Here's how the part is built. I have some questions about the finished solid (model axes, mm). A direction names the side the tool comes from. Round coordinates to 2 decimals unless told otherwise and drop trailing zeros. Order: outer loops, then holes, each group sorted by start corner. A loop starts at its lowest first (then second) coordinate and runs counter-clockwise, first axis right, second up. Notation, with made-up numbers: (-16, 19) -> (6, 19) arc R24 ccw to (6, 34) -> close; hole circle Ø11 at (-26, 69). An arc over 180 degrees is marked (long way). Use a Markdown table: item, result. Add a question column.
(1) On a 3-axis mill with a long thin cutter (end or side, diameter ignored), from which of +Z, -Z, +X, -X, +Y, -Y can I reach the whole of each face in a straight line? I mean faces 5 (the face through (25, -5, 0)), 6 (the face through (-21.07, -4.06, -10)). Say none if no direction works.
(2) I want a section at A-A, the plane y = -7. Please give me the cut outline in (x, z), then the cut area to 3 significant figures.
(3) If I drill on probe 1 along Z at (x, y) = (15.5, -5); probe 2 along X at (y, z) = (-7.75, 2); probe 3 along Y at (x, z) = (10, -6.5), over which ranges is the centre line in solid material (lowest first)?
(4) I'm going to push a flat-ended pin straight in: P1, Ø11.5, axis at x = -3.5, z = 0.5, coming from the +Y side. Where does the tip first touch, or does it pass through?
(5) I want a section at C-C, the plane z = -3. Please give me the cut outline in (x, y).
(6) Thinking about a two-plate mould opening in X: for faces 1 (the face through (0, -5, 14)), 2 (the face through (21, -4.06, -10.07)), 3 (the face through (22.5, -4, 0)), 4 (the face through (-22.861, -5.324, -11.745)), which applies, pulls with the +X half, pulls with the -X half, needs draft (parallel to the pull), parting line crosses it, or undercut?
(7) I want a section at B-B, the plane x = 7.5. Please give me the cut outline in (y, z).
from build123d import *

# Parameters (mm, degrees)
F0_W     = 45
F0_H     = 23
F1_DEPTH = 8
F2_R     = 5
F3_T     = 2.5


with BuildPart() as f1:
    # F0 (on Front) → F1 (new body)
    with BuildSketch(Plane.XZ):
        Rectangle(F0_W, F0_H)
    extrude(amount=F1_DEPTH)

    # F2
    f2_edges = [f1.edges().sort_by_distance(p)[0] for p in [
        (22.5, -4, 11.5),
        (-22.5, -4, 11.5),
        (22.5, -4, -11.5),
        (-22.5, -4, -11.5),
    ]]
    fillet(f2_edges, radius=F2_R)

    # F3
    f3_openings = [f1.faces().sort_by_distance(p)[0] for p in [
        (0, 0, 0),
    ]]
    offset(amount=F3_T, openings=f3_openings, kind=Kind.INTERSECTION)


solid = f1.part
Taken from the geometry:
| question | item | result |
|---|---|---|
| 1 | face 5 | +Z, -Z, +X, +Y, -Y |
| 1 | face 6 | +Y |
| 2 | outline | (-25, -6.5) arc R7.5 ccw to (-17.5, -14) -> (17.5, -14) arc R7.5 ccw to (25, -6.5) -> (25, 6.5) arc R7.5 ccw to (17.5, 14) -> (-17.5, 14) arc R7.5 ccw to (-25, 6.5) -> close; hole (-22.5, -6.5) arc R5 ccw to (-17.5, -11.5) -> (17.5, -11.5) arc R5 ccw to (22.5, -6.5) -> (22.5, 6.5) arc R5 ccw to (17.5, 11.5) -> (-17.5, 11.5) arc R5 ccw to (-22.5, 6.5) -> close |
| 2 | area | 338 mm2 |
| 3 | probe 1 | z = -14 to -11.5, 11.5 to 14 |
| 3 | probe 2 | x = -25 to -22.5, 22.5 to 25 |
| 3 | probe 3 | y = -10.5 to -8 |
| 4 | P1 | stops at y = -8 |
| 5 | outline | (-25, -10.5) -> (25, -10.5) -> (25, 0) -> (22.5, 0) -> (22.5, -8) -> (-22.5, -8) -> (-22.5, 0) -> (-25, 0) -> close |
| 6 | face 1 | needs draft |
| 6 | face 2 | undercut |
| 6 | face 3 | undercut |
| 6 | face 4 | pulls with the -X half |
| 7 | outline | (-10.5, -14) -> (0, -14) -> (0, -11.5) -> (-8, -11.5) -> (-8, 11.5) -> (0, 11.5) -> (0, 14) -> (-10.5, 14) -> close |
